Can you work these out from the model? Positions are in its coordinate system, mm. Give positions to 0.01 mm unless a question says otherwise; leave off trailing zeros. Order: outer loops, then holes, each group sorted by start corner. A loop starts at its lowest first (then second) coordinate and runs counter-clockwise, first axis right, second up.
```python
from build123d import *

# Parameters (mm, degrees)
F0_R     = 2.3749
F1_DEPTH = 1.905


with BuildPart() as f1:
    # F0 (on Top) → F1 (new body, symmetric)
    with BuildSketch(Plane.XY):
        with BuildLine():
            ThreePointArc((7.493, 0), (7.31599, 1.619054), (6.793324, 3.161612))
            ThreePointArc((6.793324, 3.161612), (4.813653, 5.742281), (1.926984, 7.240979))
            ThreePointArc((1.926984, 7.240979), (-0.836016, 7.446216), (-3.484713, 6.633387))
            ThreePointArc((-3.484713, 6.633387), (-5.967172, 4.531876), (-7.325286, 1.576461))
            ThreePointArc((-7.325286, 1.576461), (-0.792679, -7.450954), (7.493, 0))
        make_face()
        Circle(F0_R, mode=Mode.SUBTRACT)
    extrude(amount=F1_DEPTH, both=True)


solid = f1.part
```
1) Suppose I cut it at A-A (x = 0). Please give me the cut outline in (y, z) (3 decimals), and give its area (3 significant figures).
2) Suppose I cut it at B-B (y = 0.5). Please give me the cut outline in (x, z) (3 decimals), and give its area (3 significant figures).
3) I'm going to push a flat-ended pin straight in: pin 1 Ø1.5 at (y, z) = (-4.5, -1.5) entering from +X. Where does the tip first touch, or does it pass through?
4) Suppose I cut it at D-D (y = -2.75). Please give me the cut outline in (x, z) (3 decimals), and give its area (3 significant figures).
5) Suppose I cut it at C-C (z = 1.3). Please give me the cut outline in (x, y).
6) If I drill on line 1 (Y direction, x = 0, z = 0.2); line 2 (X direction, y = 1.5, z = 0.25); line 3 (Y direction, x = -0.5, z = -0.35), over which ranges is the centre line in solid material (lowest first)?
7) We'd pull the mould along X, two halves only. Please class faces 1 (the face through (-1.75, 1.605, -0.027)), 2 (the face through (-2, 2, 1.905)): +X half, -X half, draft (parallel to the pull), parting line (faces both ways), or undercut.
Results:
1. outline: (-7.493, -1.905) - (-2.375, -1.905) - (-2.375, 1.905) - (-7.493, 1.905) - close; (2.375, -1.905) - (7.493, -1.905) - (7.493, 1.905) - (2.375, 1.905) - close
1. area: 39.0 mm2
2. outline: (-7.476, -1.905) - (-2.322, -1.905) - (-2.322, 1.905) - (-7.476, 1.905) - close; (2.322, -1.905) - (7.476, -1.905) - (7.476, 1.905) - (2.322, 1.905) - close
2. area: 39.3 mm2
3. pin 1: stops at x = 6.49
4. outline: (-6.97, -1.905) - (6.97, -1.905) - (6.97, 1.905) - (-6.97, 1.905) - close
4. area: 53.1 mm2
5. outline: (-7.33, 1.58) arc R7.49 ccw (long way) to (7.49, 0) arc R7.49 ccw to (6.79, 3.16) arc R7.49 ccw to (1.93, 7.24) arc R7.49 ccw to (-3.48, 6.63) arc R7.49 ccw to start; hole circle Ø4.75 at (0, 0)
6. line 1: y = -7.49 to -2.37, 2.37 to 7.49
6. line 2: x = -7.34 to -1.84, 1.84 to 7.34
6. line 3: y = -7.48 to -2.32, 2.32 to 7.48
7. face 1: undercut
7. face 2: draft
